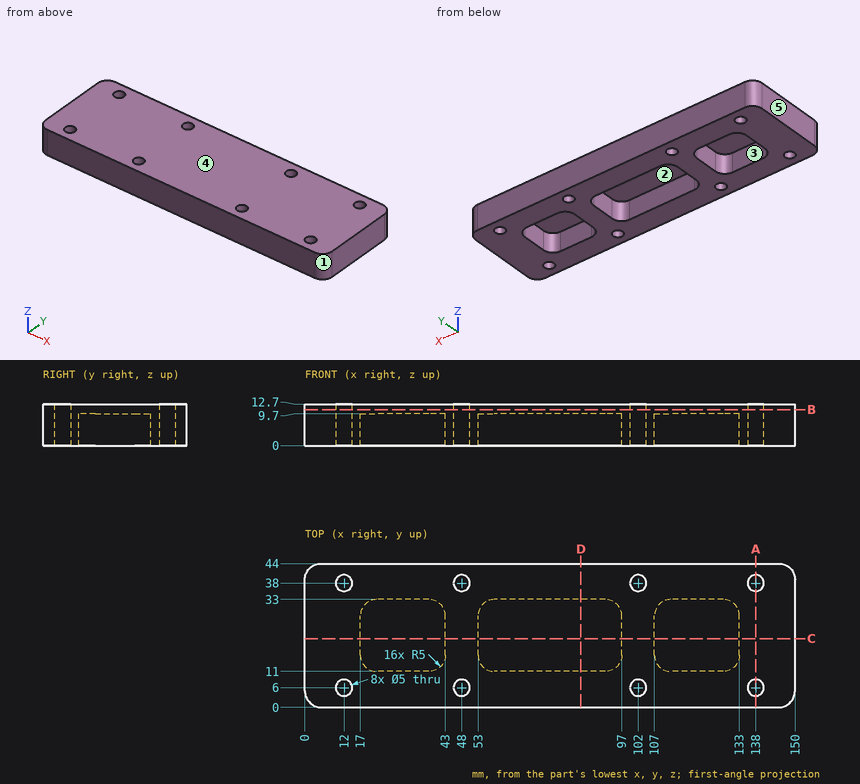
The figure shows three views and two pictorial views of one solid part (mm, origin at its lowest corner). Answer the questions. A direction names the side the tool comes from. Round coordinates to 2 decimals unless told otherwise and drop trailing zeros. Write each loop counter-clockwise with the first axis right and the second up, starting at its lowest first coordinate (ties: lowest second). Pieces come first, ordered by that corner, then holes. Notation, with made-up numbers: M 42.25,-35.5 L 73.25,-35.5 A22 ccw 73.25,-0.5 Z; hole C -1.5,21.25 d2. An arc over 180 degrees is marked long. Use a Markdown table: item, result.
1) The part is cut by section C-C (y = 21). Write down the section's boundary in (x, z), plus the area to 3 significant figures.
Answers follow:
| item | result |
|---|---|
| outline | M 0,0 L 17,0 L 17,9.7 L 43,9.7 L 43,0 L 53,0 L 53,9.7 L 97,9.7 L 97,0 L 107,0 L 107,9.7 L 133,9.7 L 133,0 L 150,0 L 150,12.7 L 0,12.7 Z |
| area | 974 mm2 |
2) A tool of negligible diameter and unlimited length cuts with its end or side. For the marked faces 1 and 2, from which of +Z, -Z, +X, -X, +Y, -Y can it reach the whole face along a straight path? Write none if from no direction.
Answers follow:
| item | result |
|---|---|
| face 1 | +Z, -Z, +X, -Y |
| face 2 | -Z |
3) The part is cut by section A-A (x = 138). Write down the section's boundary in (y, z).
Answers follow:
| item | result |
|---|---|
| outline | M 0,0 L 3.5,0 L 3.5,12.7 L 0,12.7 Z; M 8.5,0 L 35.5,0 L 35.5,12.7 L 8.5,12.7 Z; M 40.5,0 L 44,0 L 44,12.7 L 40.5,12.7 Z |
4) For a pull along X with two mould halves and no side action, classify the marked faces 3, 4 and 5 as pulls with the +X half, pulls with the -X half, needs draft (parallel to the pull), parting line crosses it, or undercut.
Answers follow:
| item | result |
|---|---|
| face 3 | undercut |
| face 4 | needs draft |
| face 5 | pulls with the -X half |
5) The part is cut by section B-B (z = 11). Give the number of separate pieces and of enclosed holes in the cut face, plus the area to 3 significant figures.
Answers follow:
| item | result |
|---|---|
| separate pieces | 1 |
| enclosed holes | 8 |
| area | 6,420 mm2 |
6) Straight lines are drawn through the part: line 1 along X through (y, z) = (23.5, 3); line 2 along Y through (x, z) = (48, 4.5); line 3 along Y through (x, z) = (72, 2). For each, find the intervals that lie inside material, in ascending order. Write a range as [from, to].
Answers follow:
| item | result |
|---|---|
| line 1 | x = [0, 17], [43, 53], [97, 107], [133, 150] |
| line 2 | y = [0, 3.5], [8.5, 35.5], [40.5, 44] |
| line 3 | y = [0, 11], [33, 44] |
7) The part is cut by section D-D (x = 84.5). Write down the section's boundary in (y, z).
Answers follow:
| item | result |
|---|---|
| outline | M 0,0 L 11,0 L 11,9.7 L 33,9.7 L 33,0 L 44,0 L 44,12.7 L 0,12.7 Z |
